The drawing under review shows one solid part. Ordinate dimensions are in mm from its lowest x, y, z. A direction names the side the tool comes from. Give positions to 0.01 mm unless a question says otherwise; leave off trailing zeros. Loops run counter-clockwise (first coordinate to the right, second up) from the corner with the lowest first, then second, coordinate; pieces in that order, holes last. Notation, with made-up numbers: M 19.5,-24.5 L 53.5,-24.5 A19 ccw 53.5,6.5 Z; hole C 24,-11.75 d10. An arc over 180 degrees is marked long. One line per item, written item: value. Start each with the question number.
Q1. We need section D-D on y = 17.5. Write out the cut boundary in (x, z).
Q2. We need section A-A on y = 38.1. Write out the cut boundary in (x, z), plus the area to 3 significant figures.
Q3. For the marked faces 5 and 6, list the 3-axis set-ups (+Z, -Z, +X, -X, +Y, -Y) from which the entire face can be reached by the end or side of a thin tool; tool diameter is ignored.
Q4. For pin 1 (1.9 mm diameter, centred on x = 75.5, y = 2.5, fed in from +Z), flat-tipped, find the tip position at first contact; note if it passes through.
Q5. Mouldability with a two-part tool opening along Y and no side actions: class the marked faces 1, 2, 3 and 4 as released by +Y, released by -Y, zero draft, split by the parting line, or undercut.
Q6. We need section C-C on x = 88. Write out the cut boundary in (y, z).
Q7. We need section B-B on z = 22. Write out the cut boundary in (x, y).
Q8. To check wall thickness, follow line 1 along Y through (x, z) = (12.5, 3); line 2 along Z through (x, y) = (3.5, 38.1); line 3 along X through (y, z) = (37, 56.5). State the ranges of each line that lie inside material, in increasing order. Write a range as from..to.
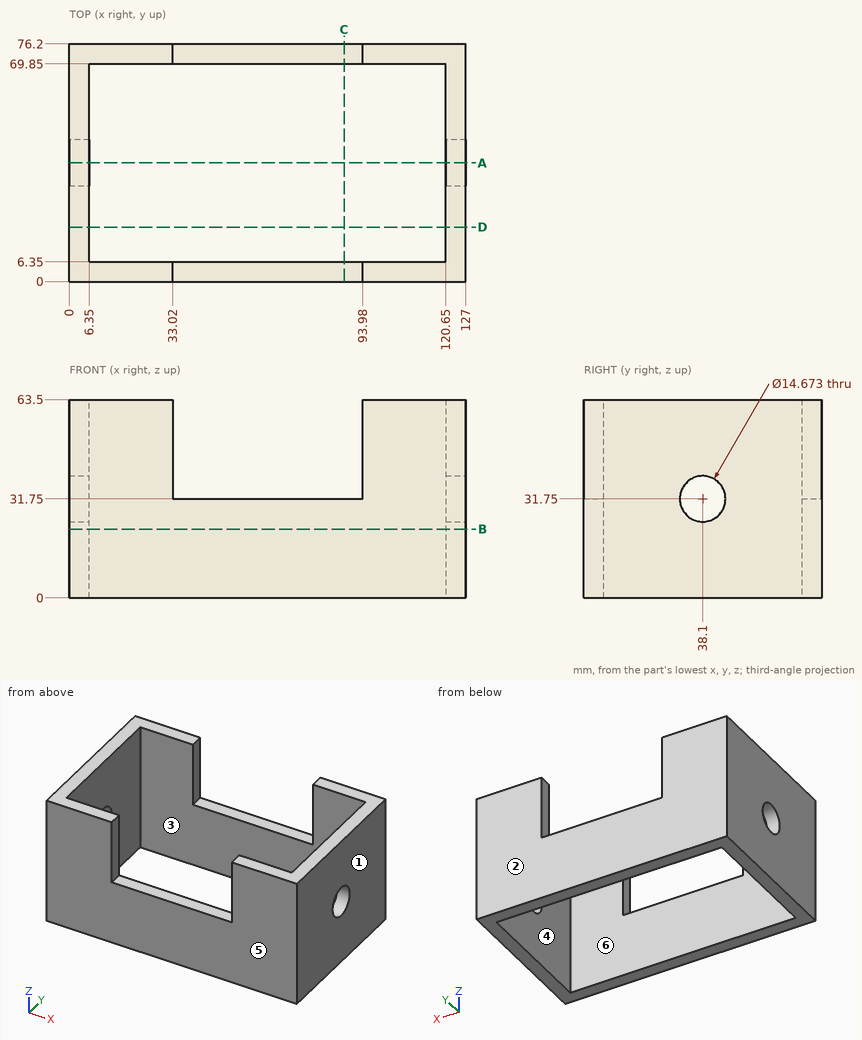
Solved:
1. outline: M 0,0 L 6.35,0 L 6.35,63.5 L 0,63.5 Z; M 120.65,0 L 127,0 L 127,63.5 L 120.65,63.5 Z
2. outline: M 0,0 L 6.35,0 L 6.35,24.41 L 0,24.41 Z; M 0,39.09 L 6.35,39.09 L 6.35,63.5 L 0,63.5 Z; M 120.65,0 L 127,0 L 127,24.41 L 120.65,24.41 Z; M 120.65,39.09 L 127,39.09 L 127,63.5 L 120.65,63.5 Z
2. area: 620 mm2
3. face 5: +Z, -Z, +X, -X, -Y
3. face 6: +Z, -Z
4. pin 1: z = 31.75
5. face 1: zero draft
5. face 2: released by +Y
5. face 3: undercut
5. face 4: undercut
6. outline: M 0,0 L 6.35,0 L 6.35,31.75 L 0,31.75 Z; M 69.85,0 L 76.2,0 L 76.2,31.75 L 69.85,31.75 Z
7. outline: M 0,0 L 127,0 L 127,76.2 L 0,76.2 Z; hole M 6.35,6.35 L 120.65,6.35 L 120.65,69.85 L 6.35,69.85 Z
8. line 1: 0..6.35, 69.85..76.2
8. line 2: 0..24.41, 39.09..63.5
8. line 3: 0..6.35, 120.65..127
